Work out the finished part from the listing and answer in its coordinate system (mm). Give positions to 0.01 mm unless a question says otherwise; leave off trailing zeros. Loops run counter-clockwise (first coordinate to the right, second up) from the corner with the lowest first, then second, coordinate; pieces in that order, holes last. Notation, with made-up numbers: M 14.25,29 L 46.25,29 A26 ccw 46.25,66 Z; hole C 34,14 d2. An arc over 180 degrees is marked long. Use a Markdown table: item, result.
Autodesk Inventor part; units mm, degrees
ref_plane "YZ Plane" through (0, 0, 0) normal (1, 0, 0) x (0, 1, 0)
ref_plane "XZ Plane" through (0, 0, 0) normal (0, 1, 0) x (-1, 0, 0)
ref_plane "XY Plane" through (0, 0, 0) normal (0, 0, 1) x (1, 0, 0)
sketch "スケッチ1" plane through (0, 0, 0) normal (0, 0, 1) x (1, 0, 0)
  point P0 (0, 0)
sketch "スケッチ2" plane through (0, 0, 0) normal (0, 0, 1) x (1, 0, 0)
  line L0 (72.5, -37.5) -> (-72.5, -37.5)
  line L1 (-72.5, -37.5) -> (-72.5, 37.5)
  line L2 (-72.5, 37.5) -> (72.5, 37.5)
  line L3 (72.5, 37.5) -> (72.5, -37.5)
  line L4 (72.5, -37.5) -> (-72.5, 37.5) construction
  line L5 (-72.5, -37.5) -> (72.5, 37.5) construction
  line L6 (67.5, 32.5) -> (-67.5, 32.5)
  line L7 (-67.5, 32.5) -> (-67.5, -32.5)
  line L8 (-67.5, -32.5) -> (67.5, -32.5)
  line L9 (67.5, -32.5) -> (67.5, 32.5)
  line L10 (-67.5, 32.5) -> (-67.5, 12.5) construction
  line L11 (-69.1, 32.5) -> (-69.1, 12.5)
  line L12 (-65.9, 12.5) -> (-65.9, 32.5)
  arc A0 (-65.9, 32.5) -> (-69.1, 32.5) centre (-67.5, 32.5) ccw
  arc A1 (-69.1, 12.5) -> (-65.9, 12.5) centre (-67.5, 12.5) ccw
  line L13 (-67.5, 32.5) -> (-47.5, 32.5) construction
  line L14 (-67.5, -32.5) -> (-67.5, -12.5) construction
  line L15 (-65.9, -32.5) -> (-65.9, -12.5)
  line L16 (-69.1, -12.5) -> (-69.1, -32.5)
  arc A2 (-69.1, -32.5) -> (-65.9, -32.5) centre (-67.5, -32.5) ccw
  arc A3 (-65.9, -12.5) -> (-69.1, -12.5) centre (-67.5, -12.5) ccw
  line L17 (-67.5, -32.5) -> (-47.5, -32.5) construction
  line L18 (67.5, 32.5) -> (67.5, 12.5) construction
  line L19 (65.9, 32.5) -> (65.9, 12.5)
  line L20 (69.1, 12.5) -> (69.1, 32.5)
  arc A4 (69.1, 32.5) -> (65.9, 32.5) centre (67.5, 32.5) ccw
  arc A5 (65.9, 12.5) -> (69.1, 12.5) centre (67.5, 12.5) ccw
  line L21 (67.5, 32.5) -> (87.5, 32.5) construction
  line L22 (67.5, -32.5) -> (67.5, -12.5) construction
  line L23 (69.1, -32.5) -> (69.1, -12.5)
  line L24 (65.9, -12.5) -> (65.9, -32.5)
  arc A6 (65.9, -32.5) -> (69.1, -32.5) centre (67.5, -32.5) ccw
  arc A7 (69.1, -12.5) -> (65.9, -12.5) centre (67.5, -12.5) ccw
  line L25 (67.5, -32.5) -> (87.5, -32.5) construction
  line L26 (-72.5, -17) -> (72.5, -17)
  circle A8 centre (0, -17) radius 9
  circle A9 centre (0, -17) radius 39
  line L27 (0, 37.5) -> (0, -37.5)
  line L28 (-57.5, 37.5) -> (60, 37.5)
  line L29 (60, 37.5) -> (60, 32.5)
  line L30 (60, 32.5) -> (-60, 32.5)
  circle A10 centre (0, -155) radius 120
  circle A11 centre (-67.5, 32.5) radius 1.6
  circle A12 centre (-67.5, -12.5) radius 1.6
  circle A13 centre (67.5, 32.5) radius 1.6
  circle A14 centre (67.5, -12.5) radius 1.6
  circle A15 centre (-57.5, -17) radius 1.6
  circle A16 centre (-57.5, 17) radius 1.6
  circle A17 centre (57.5, -17) radius 1.6
  circle A18 centre (57.5, 17) radius 1.6
  line L31 (0, -32.5) -> (-72.5, -19.1)
  line L32 (0, -32.5) -> (72.5, -19.1)
  line L33 (67.5, -19.1) -> (-67.5, -19.1)
  circle A19 centre (-37.5, 32.5) radius 1.6
  circle A20 centre (-27.5, 17) radius 1.6
  circle A21 centre (-37.5, -12.5) radius 1.6
  circle A22 centre (-27.5, -17) radius 1.6
  line L34 (-42.5, 37.5) -> (-42.5, -37.5)
  point P0 (0, 0)
  point P1 (-67.5, 22.5)
  point P2 (67.5, 22.5)
  point P3 (60, 37.5)
  point P4 (-24.367, -37.5)
  point P5 (24.367, -37.5)
  point P6 (-65.9, 32.5)
  point P7 (69.1, -12.5)
  point P8 (65.9, 32.5)
  point P9 (69.1, 32.5)
  point P10 (-65.9, -12.5)
  point P11 (-35.7876, -32.5)
  point P12 (35.7876, -32.5)
  point P13 (0, 0)
  point P14 (72.5, -19.1)
  point P15 (-65.9, 32.5)
  point P16 (65.9, 32.5)
  point P17 (80, 36.6)
  point P18 (-65.9, 32.5)
  point P19 (65.9, 32.5)
  point P20 (67.5, 30.9)
  point P21 (-67.5, 30.9)
  point P22 (67.5, 10.9)
  point P23 (-67.5, 10.9)
  point P24 (-33.1776, -37.5)
  point P25 (33.1776, -37.5)
  point P26 (-42.5, 37.5)
  point P27 (-42.5, -24.6448)
  dimension "d0" = 145
  dimension "d1" = 75
  dimension "d21" = 5
  dimension "d22" = 20
  dimension "d23" = 90
  dimension "d24" = 3.2
  dimension "d25" = 20
  dimension "d26" = 90
  dimension "d27" = 3.2
  dimension "d28" = 20
  dimension "d29" = 90
  dimension "d30" = 3.2
  dimension "d31" = 20
  dimension "d32" = 90
  dimension "d33" = 3.2
  dimension "d36" = 20.5
  dimension "d37" = 18
  dimension "d38" = 78
  dimension "d42" = 120
  dimension "d43" = 60
  dimension "d45" = 240
  dimension "d46" = 138
  dimension "d47" = 3.2
  dimension "d48" = 10
  dimension "d49" = 3.2
  dimension "d50" = 10
  dimension "d51" = 17
  dimension "d52" = 17
  dimension "d54" = 5
  dimension "d57" = 30
  dimension "d62" = 30
extrude "押し出し1" add sketch "スケッチ2" along normal blind 3 contours L34 L33 A9 L31 | L31 A9 L33 A8 L27 | L27 A8 L33 A9 L32 | L34 L26 A9 L33 | A9 L33 L24 L32 | A9 L26 A22 A8 L33 | L34 L6 A19 L27 A9 A21 L26 | A8 L26 A9 L33 | A9 L26 A17 L24 L33 | L24 L33 L9 L32 | A9 A21 L27 A8 L26 A22 | L34 L2 L27 L6 A19 | A8 L27 A9 L26 | A9 L27 L6 L19 A5 L9 A7 L24 L26 A17 | L24 L26 L9 L33 | L9 L26 L23 L32 | L32 L23 L26 L3 | L2 L29 L6 L27 | L24 A14 L9 L26 | L26 L23 A7 L9 A5 L20 A4 L6 L29 L2 L3 | L26 L9 A14 L23 | A13 L9 A5 L19 | L9 A13 L20 A5
fillet "フィレット1" radius 5 5 edges at (72.5, 37.5, 1.5) (72.5, -19.1, 1.5) (0, -32.5, 1.5) (-42.5, -24.6448, 1.5) (-42.5, 37.5, 1.5)
sketch "スケッチ4" plane through (0, 0, 0) normal (0, 0, -1) x (-1, 0, 0)
  circle A0 centre (-57.5, -17) radius 1.6
  circle A1 centre (-57.5, 17) radius 1.6
  circle A2 centre (-67.5, 32.5) radius 1.6
  circle A3 centre (-67.5, -12.5) radius 1.6
  line L0 (-72.5, -14.9395) -> (-72.5, 32.5)
  line L1 (-67.5, 37.5) -> (37.5, 37.5)
  arc A4 (-67.5, 37.5) -> (-72.5, 32.5) centre (-67.5, 32.5) ccw
  line L2 (42.5, 32.5) -> (42.5, -20.4843)
  arc A5 (-0.9087, -32.332) -> (0.9087, -32.332) centre (0, -27.4153) ccw
  line L3 (38.4087, -25.401) -> (0.9087, -32.332)
  arc A6 (-72.5, -14.9395) -> (-68.4087, -19.8562) centre (-67.5, -14.9395) ccw
  line L4 (-0.9087, -32.332) -> (-68.4087, -19.8562)
  arc A7 (42.5, 32.5) -> (37.5, 37.5) centre (37.5, 32.5) ccw
  arc A8 (38.4087, -25.401) -> (42.5, -20.4843) centre (37.5, -20.4843) ccw
  point P0 (0, 0)
equation "\"d25\" = d22"
equation "\"d27\" = d24"
equation "\"d28\" = d22"
equation "\"d30\" = d24"
equation "\"d31\" = d22"
equation "\"d33\" = d24"
equation "\"d43\" = 0.5 * d42"
properties part number "small_plate_nomotor"
(1) A cutting plane is placed at B-B (x = 57.5). Write down the section's boundary in (y, z), and give its area (3 significant figures).
Entries:
| item | result |
|---|---|
| outline | M -21.87,0 L -18.6,0 L -18.6,3 L -21.87,3 Z; M -15.4,0 L 15.4,0 L 15.4,3 L -15.4,3 Z; M 18.6,0 L 37.5,0 L 37.5,3 L 18.6,3 Z |
| area | 159 mm² |
(2) A cutting plane is placed at C-C (y = -12.5). Write down the section's boundary in (x, z), and give its area (3 significant figures).
Entries:
| item | result |
|---|---|
| outline | M -42.5,0 L -39.1,0 L -39.1,3 L -42.5,3 Z; M -35.9,0 L -7.79,0 L -7.79,3 L -35.9,3 Z; M 7.79,0 L 65.9,0 L 65.9,3 L 7.79,3 Z; M 69.1,0 L 72.5,0 L 72.5,3 L 69.1,3 Z |
| area | 279 mm² |
(3) A cutting plane is placed at A-A (z = 1.85). Count the separate pieces of the cut face and the enclosed holes in it, and give its area (3 significant figures).
Entries:
| item | result |
|---|---|
| separate pieces | 1 |
| enclosed holes | 9 |
| area | 7,060 mm² |
(4) A cutting plane is placed at D-D (x = 5). Write down the section's boundary in (y, z), and give its area (3 significant figures).
Entries:
| item | result |
|---|---|
| outline | M -31.58,0 L -24.48,0 L -24.48,3 L -31.58,3 Z; M -9.52,0 L 37.5,0 L 37.5,3 L -9.52,3 Z |
| area | 162 mm² |
(5) The mould has two halves that part along X. Classify faces 1 (the flat face through (14, 3, 0)), 2 (the cylindrical face through (-28.68, 15.92, 1.48)), 3 (the cylindrical face through (71.07, 36, 1.52)), 4 (the flat face through (-42.5, 6, 1)): released by +X, released by -X, zero draft, split by the parting line, or undercut.
Entries:
| item | result |
|---|---|
| face 1 | zero draft |
| face 2 | undercut |
| face 3 | released by +X |
| face 4 | released by -X |
(6) Consider probe 1 along Y at (x, z) = (0, 0.95); probe 2 along X at (y, z) = (-12.5, 1.7); probe 3 along X at (y, z) = (-17, 1.7). Determine where each line is inside the solid, lowest interval first. Write a range as [from, to].
Entries:
| item | result |
|---|---|
| probe 1 | y = [-32.42, -26], [-8, 37.5] |
| probe 2 | x = [-42.5, -39.1], [-35.9, -7.79], [7.79, 65.9], [69.1, 72.5] |
| probe 3 | x = [-42.5, -29.1], [-25.9, -9], [9, 55.9], [59.1, 72.06] |
(7) Given P1, Ø5, axis at x = -37.5, y = -12.5, coming from the -Z side, flat-ended and moving along its own axis, determine where the tip first touches the part or whether it passes through.
Entries:
| item | result |
|---|---|
| P1 | stops at z = 0 |
